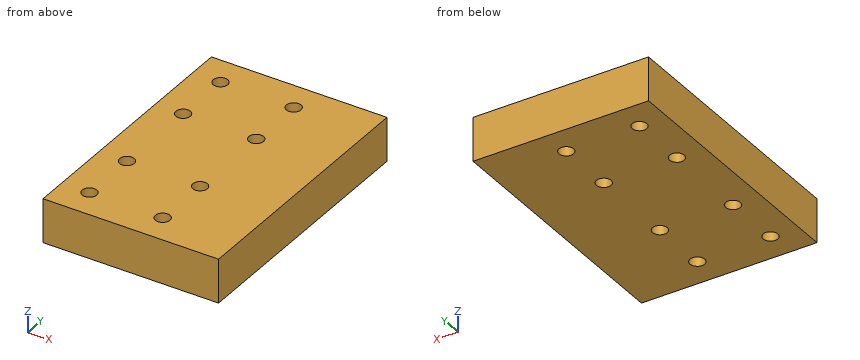
```python
from build123d import *

# Parameters (mm, degrees)
ESQUISSE1_W                  = 60
ESQUISSE1_H                  = 90
BOSS_EXTRU_1_DEPTH           = 15
ENL_V_MAT_EXTRU_1_DEPTH      = 110.201648339
ENL_V_MAT_EXTRU_1_DEPTH_BACK = 110.201648339
ESQUISSE2_R                  = 2.5


with BuildPart() as part:
    # Esquisse1 → Boss.-Extru.1 (new body)
    with BuildSketch(Plane.XY):
        with Locations((30, 45)):
            Rectangle(ESQUISSE1_W, ESQUISSE1_H)
    extrude(amount=BOSS_EXTRU_1_DEPTH)

    # Esquisse2 → Enlèv. mat.-Extru.1 (cut, two sides: drawn at the far end of the back side and taken through both)
    with BuildSketch(Plane.XY.offset(15).offset(-ENL_V_MAT_EXTRU_1_DEPTH_BACK)):
        with Locations((9.5, 10)):
            Circle(ESQUISSE2_R)
        with Locations(Location((34.5, 10, 0), (0, 0, 180))):
            Circle(ESQUISSE2_R)
        with Locations((34.5, 30)):
            Circle(ESQUISSE2_R)
        with Locations(Location((9.5, 30, 0), (0, 0, 180))):
            Circle(ESQUISSE2_R)
        with Locations((9.5, 60)):
            Circle(ESQUISSE2_R)
        with Locations(Location((34.5, 60, 0), (0, 0, 180))):
            Circle(ESQUISSE2_R)
        with Locations((34.5, 80)):
            Circle(ESQUISSE2_R)
        with Locations(Location((9.5, 80, 0), (0, 0, 180))):
            Circle(ESQUISSE2_R)
    extrude(amount=ENL_V_MAT_EXTRU_1_DEPTH + ENL_V_MAT_EXTRU_1_DEPTH_BACK, mode=Mode.SUBTRACT)


solid = part.part
```
Input: part model. Units: mm. Frame: model coordinates. Give positions to 0.01 mm unless a question says otherwise; leave off trailing zeros. Order: outer loops, then holes, each group sorted by start corner. A loop starts at its lowest first (then second) coordinate and runs counter-clockwise, first axis right, second up. Notation, with made-up numbers: M 39.25,-11.75 L 81.25,-11.75 A4 ccw 81.25,-4.75 Z; hole C -6,65.5 d6. An arc over 180 degrees is marked long. One line per question, with ' | ' between items. Start each with the question number.
1. Section query A-A (y = 30). Return the cut outline in (x, z).
2. Section query D-D (y = 11). Return the cut outline in (x, z), and give its area (3 significant figures).
3. Section query B-B (z = 8.5). Count the separate pieces of the cut face and the enclosed holes in it, and give its area (3 significant figures).
4. Section query C-C (x = 9.5). Return the cut outline in (y, z), and give its area (3 significant figures).
5. Material intervals for probe 1 along Y at (x, z) = (9.5, 5.5); probe 2 along X at (y, z) = (61, 14); probe 3 along X at (y, z) = (59.5, 6.75), sorted ascending. Write a range as [from, to].
Here are the results:
1) outline: M 0,0 L 7,0 L 7,15 L 0,15 Z; M 12,0 L 32,0 L 32,15 L 12,15 Z; M 37,0 L 60,0 L 60,15 L 37,15 Z
2) outline: M 0,0 L 7.21,0 L 7.21,15 L 0,15 Z; M 11.79,0 L 32.21,0 L 32.21,15 L 11.79,15 Z; M 36.79,0 L 60,0 L 60,15 L 36.79,15 Z | area: 763 mm²
3) separate pieces: 1 | enclosed holes: 8 | area: 5,240 mm²
4) outline: M 0,0 L 7.5,0 L 7.5,15 L 0,15 Z; M 12.5,0 L 27.5,0 L 27.5,15 L 12.5,15 Z; M 32.5,0 L 57.5,0 L 57.5,15 L 32.5,15 Z; M 62.5,0 L 77.5,0 L 77.5,15 L 62.5,15 Z; M 82.5,0 L 90,0 L 90,15 L 82.5,15 Z | area: 1,050 mm²
5) probe 1: [0, 7.5], [12.5, 27.5], [32.5, 57.5], [62.5, 77.5], [82.5, 90] | probe 2: [0, 7.21], [11.79, 32.21], [36.79, 60] | probe 3: [0, 7.05], [11.95, 32.05], [36.95, 60]
